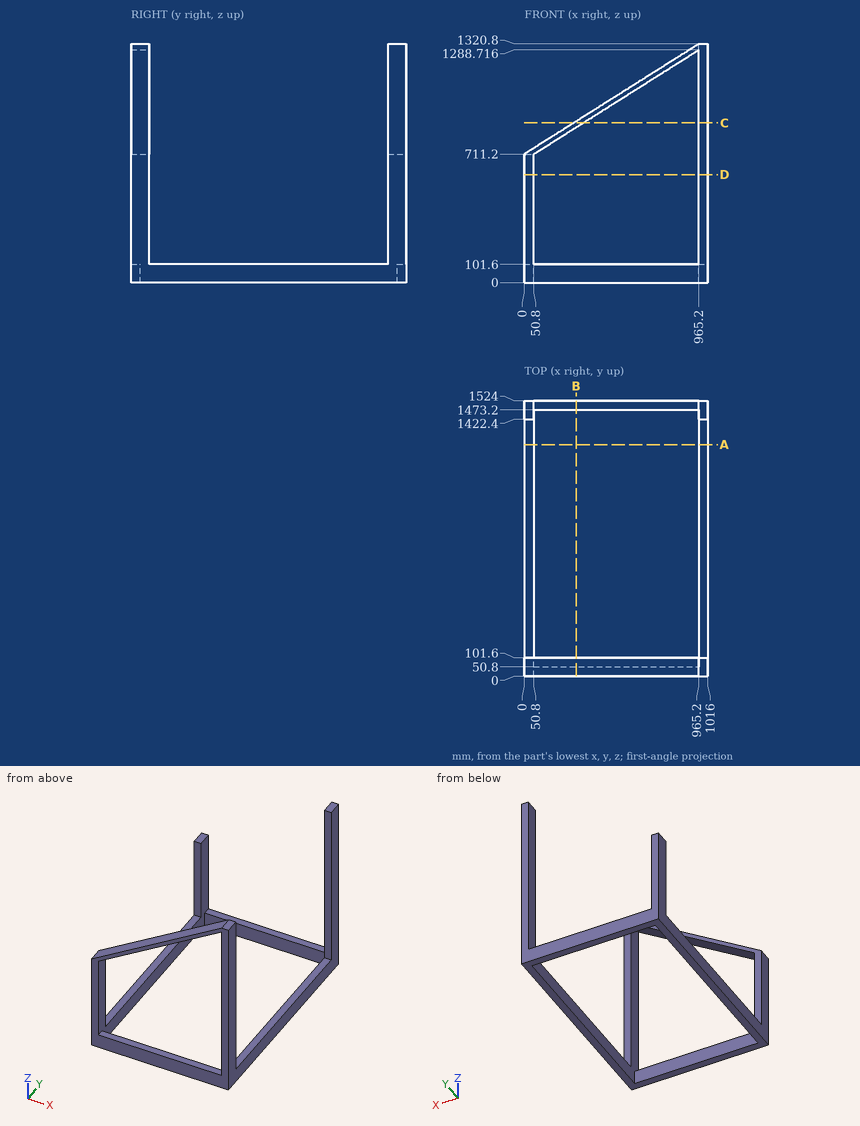
Geometry check sheet. Reference: drawing and pictorial views, mm from the part's lowest x, y, z. Coordinates: 2 decimals unless noted, no trailing zeros. Order: outer loops, then holes, each group sorted by start corner. A loop starts at its lowest first (then second) coordinate and runs counter-clockwise, first axis right, second up. Notation, with made-up numbers: (-35, -7.5) -> (-21, -7.5) arc R22 cw to (-21, 23.5) -> close; hole circle Ø11 at (60, -38.75). An arc over 180 degrees is marked (long way). Use CSV: the item, a comma, the result in double quotes. Start each with the question number.
Q1. Section check C-C, the plane z = 884.5. Record the cut outline in (x, y).
Q2. Section check B-B, the plane x = 286.5. Record the cut outline in (y, z), and give its area (3 significant figures).
Q3. Section check D-D, the plane z = 597.5. Record the cut outline in (x, y).
Q4. Section check A-A, the plane y = 1280. Record the cut outline in (x, z), and give its area (3 significant figures).
Q5. Thickness scan on line 1 along X through (y, z) = (1459, 433.5); line 2 along Z through (x, y) = (904, 61.5). Record the ranges inside material, lowest first.
Returned:
1,outline,"(274.39, 0) -> (325.19, 0) -> (325.19, 101.6) -> (274.39, 101.6) -> close; (965.2, 0) -> (1016, 0) -> (1016, 101.6) -> (965.2, 101.6) -> close; (965.2, 1422.4) -> (1016, 1422.4) -> (1016, 1524) -> (965.2, 1524) -> close"
2,outline,"(0, 0) -> (50.8, 0) -> (50.8, 101.6) -> (0, 101.6) -> close; (0, 860.06) -> (101.6, 860.06) -> (101.6, 892.15) -> (0, 892.15) -> close; (1473.2, 0) -> (1524, 0) -> (1524, 101.6) -> (1473.2, 101.6) -> close"
2,area,"13,600 mm^2"
3,outline,"(0, 0) -> (50.8, 0) -> (50.8, 101.6) -> (0, 101.6) -> close; (0, 1422.4) -> (50.8, 1422.4) -> (50.8, 1524) -> (0, 1524) -> close; (965.2, 0) -> (1016, 0) -> (1016, 101.6) -> (965.2, 101.6) -> close; (965.2, 1422.4) -> (1016, 1422.4) -> (1016, 1524) -> (965.2, 1524) -> close"
4,outline,"(0, 0) -> (50.8, 0) -> (50.8, 101.6) -> (0, 101.6) -> close; (965.2, 0) -> (1016, 0) -> (1016, 101.6) -> (965.2, 101.6) -> close"
4,area,"10,300 mm^2"
5,line 1,"x = 0 to 50.8, 965.2 to 1016"
5,line 2,"z = 1250.06 to 1282.15"
